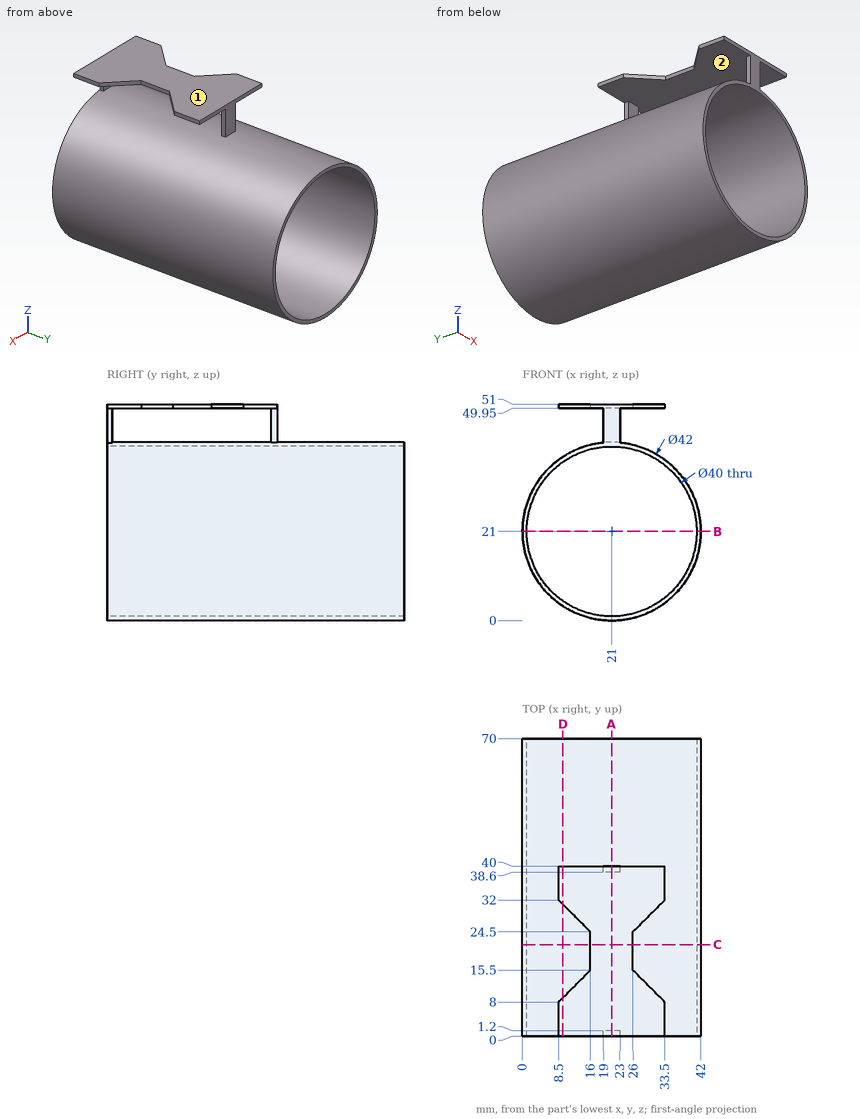
Here's the drawing with two shaded views (mm, measured from the low corner). I have some questions. Coordinates: 2 decimals unless noted, no trailing zeros. Write each loop counter-clockwise with the first axis right and the second up, starting at its lowest first coordinate (ties: lowest second). Pieces come first, ordered by that corner, then holes. Notation, with made-up numbers: M 50.25,16 L 98.25,16 A30 ccw 98.25,50 Z; hole C 63,8.5 d6. An arc over 180 degrees is marked long. Answer as CSV lines item,"result". Start each with the question number.
1) I want a section at C-C, the plane y = 21.5. Please give me the cut outline in (x, z), and give its area (3 significant figures).
2) We'd pull the mould along Y, two halves only. Please class the marked faces 1 and 2: +Y half, -Y half, draft (parallel to the pull), parting line (faces both ways), or undercut.
3) Please list where these lines run through material, in increasing order: line 1 (Y direction, x = 22.5, z = 42); line 2 (Z direction, x = 18, y = 13); line 3 (X direction, y = 19, z = 20.5). Write a range as from..to.
4) I want a section at B-B, the plane z = 21. Please give me the cut outline in (x, y), and give its area (3 significant figures).
5) I want a section at D-D, the plane x = 9.5. Please give me the cut outline in (y, z).
6) I want a section at A-A, the plane x = 21. Please give me the cut outline in (y, z), and give its area (3 significant figures).
7) For P1, Ø8, axis at y = 12.5, z = 34.5, coming from the -X side; P2, Ø12.5, axis at x = 23.5, y = 22.5, coming from the -Z side; P3, Ø1.3, axis at y = 1, z = 44.5, coming from the +X side; P4, Ø1.2, axis at y = 18, z = 50.5, coming from the -X side, each with a flat end and sliding along its axis, tell me the tip position at first contact or that it passes through.
Data:
1,outline,"C 21,21 d42; M 16,49.95 L 26,49.95 L 26,51 L 16,51 Z; hole C 21,21 d40"
1,area,"139 mm^2"
2,face 1,"draft"
2,face 2,"undercut"
3,line 1,"y = 0..1.2, 38.6..40"
3,line 2,"z = 0.22..1.23, 40.77..41.78, 49.95..51"
3,line 3,"x = 0.01..1.01, 40.99..41.99"
4,outline,"M 0,0 L 1,0 L 1,70 L 0,70 Z; M 41,0 L 42,0 L 42,70 L 41,70 Z"
4,area,"140 mm^2"
5,outline,"M 0,3.43 L 70,3.43 L 70,4.64 L 0,4.64 Z; M 0,37.36 L 70,37.36 L 70,38.57 L 0,38.57 Z; M 0,49.95 L 9,49.95 L 9,51 L 0,51 Z; M 31,49.95 L 40,49.95 L 40,51 L 31,51 Z"
6,outline,"M 0,0 L 70,0 L 70,1 L 0,1 Z; M 0,41 L 70,41 L 70,42 L 40,42 L 40,51 L 0,51 Z; hole M 1.2,42 L 38.6,42 L 38.6,49.95 L 1.2,49.95 Z"
6,area,"203 mm^2"
7,P1,"stops at x = 2.27"
7,P2,"stops at z = 0"
7,P3,"stops at x = 23"
7,P4,"stops at x = 16"
